The model under review builds one solid part; all positions refer to its coordinate system, in mm. Face numbers are marked on the shaded views. A direction names the side the tool comes from. Round coordinates to 2 decimals unless told otherwise and drop trailing zeros. Order: outer loops, then holes, each group sorted by start corner. A loop starts at its lowest first (then second) coordinate and runs counter-clockwise, first axis right, second up.
1) Clearance check with flat-ended pins moving along their axes: P1, Ø6, axis at x = -37.5, y = 103, coming from the +Z side; P2, Ø8, axis at x = 37.5, y = 103, coming from the +Z side; P3, Ø3, axis at x = 3, z = 33, coming from the -Y side. State where each tip first meets the part, or that it passes through.
2) To check wall thickness, follow L1, parallel to X at y = 8, z = 33.1; L2, parallel to X at y = 103, z = 18; L3, parallel to X at y = 132, z = 15.5. State the ranges of each line that lie inside material, in increasing order.
3) Consider section C-C (z = 7). Give the number of separate pieces and of enclosed holes in the cut face, then the cut area to 3 significant figures.
4) Machinability: for the marked faces 1, 2 and 3, which of the approach directions +Z, -Z, +X, -X, +Y, -Y give a long, thin tool a straight path to every point of the face, cutting with its end or side? Answer none if there is none.
5) Consider section A-A (x = 0). Give the boundary of the cut face in (y, z).
6) Consider section D-D (y = 118). Give the boundary of the cut face in (x, z).
7) Mouldability with a two-part tool opening along Y and no side actions: class the marked faces 4, 5, 6 and 7 as pulls with the +Y half, pulls with the -Y half, needs draft (parallel to the pull), parting line crosses it, or undercut.
8) Consider section B-B (y = 188). Give the boundary of the cut face in (x, z), then the cut area to 3 significant figures.
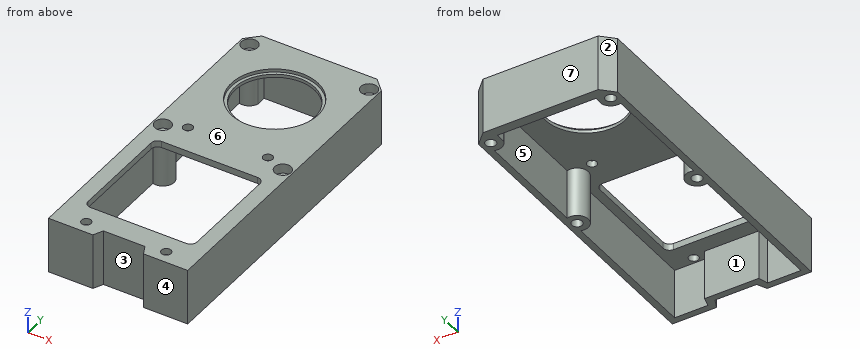
from build123d import *

# Parameters (mm, degrees)
SKETCH_R        = 3.25
SKETCH_R_2      = 3
SKETCH_R_3      = 25
PAD_DEPTH       = 35
POCKET_DEPTH    = 31
SKETCH003_R     = 5.1
POCKET001_DEPTH = 6
SKETCH004_R     = 27
POCKET002_DEPTH = 2


with BuildPart() as part:
    # Sketch → Pad (new body)
    with BuildSketch(Plane.XY):
        Polygon((-43.5, 190.5), (-43.5, 0), (-15.797846, 0), (-13, 6), (13, 6), (15.797846, 0), (43.5, 0), (43.5, 190.5), (36, 198), (-36, 198), align=None)
        with Locations((-37.5, 188)):
            Circle(SKETCH_R, mode=Mode.SUBTRACT)
        with Locations((37.5, 188)):
            Circle(SKETCH_R, mode=Mode.SUBTRACT)
        with Locations((-25, 108)):
            Circle(SKETCH_R_2, mode=Mode.SUBTRACT)
        with Locations((25, 108)):
            Circle(SKETCH_R_2, mode=Mode.SUBTRACT)
        with Locations((37.5, 103)):
            Circle(SKETCH_R, mode=Mode.SUBTRACT)
        with Locations((-37.5, 103)):
            Circle(SKETCH_R, mode=Mode.SUBTRACT)
        with Locations((-25, 8)):
            Circle(SKETCH_R_2, mode=Mode.SUBTRACT)
        with Locations((25, 8)):
            Circle(SKETCH_R_2, mode=Mode.SUBTRACT)
        with Locations((0, 154)):
            Circle(SKETCH_R_3, mode=Mode.SUBTRACT)
        with BuildLine():
            ThreePointArc((-30, 90), (-32.828431, 88.828423), (-34, 85.999989))
            Line((-34, 24), (-34, 85.999989))
            ThreePointArc((-34, 24), (-32.828427, 21.171573), (-30, 20))
            Line((-30, 20), (30, 20))
            ThreePointArc((30, 20), (32.828427, 21.171573), (34, 24))
            Line((34, 85.999989), (34, 24))
            ThreePointArc((34, 85.999989), (32.828431, 88.828424), (29.999999, 90))
            Line((-30, 90), (29.999999, 90))
        make_face(mode=Mode.SUBTRACT)
    extrude(amount=PAD_DEPTH)

    # Sketch002 → Pocket (cut)
    with BuildSketch(Plane(origin=(0, 0, 0), x_dir=(1, 0, 0), z_dir=(0, 0, -1))):
        with BuildLine():
            Line((-39.5, -96.291796), (-39.5, -4))
            Line((-39.5, -4), (-18.607695, -4))
            Line((-18.607695, -4), (-17, -10))
            Line((-17, -10), (17, -10))
            Line((17, -10), (18.607695, -4))
            Line((18.607695, -4), (39.5, -4))
            Line((39.5, -4), (39.5, -96.291796))
            ThreePointArc((39.5, -96.291796), (30.5, -103), (39.5, -109.708204))
            Line((39.5, -109.708204), (39.5, -181.291796))
            ThreePointArc((39.5, -181.291796), (34.170797, -181.84237), (30.791796, -186))
            Line((30.791796, -192), (30.791796, -186))
            Line((-30.791796, -192), (30.791796, -192))
            Line((-30.791796, -186), (-30.791796, -192))
            ThreePointArc((-30.791796, -186), (-34.170797, -181.84237), (-39.5, -181.291796))
            Line((-39.5, -109.708204), (-39.5, -181.291796))
            ThreePointArc((-39.5, -109.708204), (-30.5, -103), (-39.5, -96.291796))
        make_face()
    extrude(amount=-POCKET_DEPTH, mode=Mode.SUBTRACT)

    # Sketch003 → Pocket001 (cut)
    with BuildSketch(Plane.XY.offset(35)):
        with Locations((-37.371348, 188)):
            Circle(SKETCH003_R)
        with Locations((37.371348, 188)):
            Circle(SKETCH003_R)
        with Locations((-37.5, 103)):
            Circle(SKETCH003_R)
        with Locations((37.5, 103)):
            Circle(SKETCH003_R)
    extrude(amount=-POCKET001_DEPTH, mode=Mode.SUBTRACT)

    # Sketch004 → Pocket002 (cut)
    with BuildSketch(Plane.XY.offset(35)):
        with Locations((0, 154)):
            Circle(SKETCH004_R)
    extrude(amount=-POCKET002_DEPTH, mode=Mode.SUBTRACT)


solid = part.part
Answer below:
1. P1: passes through
1. P2: stops at z = 29
1. P3: stops at y = 6
2. L1: x = -43.5 to -28, -22 to 22, 28 to 43.5
2. L2: x = -43.5 to -40.75, -34.25 to -30.5, 30.5 to 34.25, 40.75 to 43.5
2. L3: x = -43.5 to -39.5, 39.5 to 43.5
3. separate pieces: 1
3. enclosed holes: 5
3. area: 2,610 mm2
4. face 1: -Z
4. face 2: +Z, -Z, -X, +Y
4. face 3: +Z, -Z, -Y
5. outline: (6, 0) - (10, 0) - (10, 31) - (20, 31) - (20, 35) - (6, 35) - close; (90, 31) - (129, 31) - (129, 33) - (127, 33) - (127, 35) - (90, 35) - close; (179, 31) - (192, 31) - (192, 0) - (198, 0) - (198, 35) - (181, 35) - (181, 33) - (179, 33) - close
6. outline: (-43.5, 0) - (-39.5, 0) - (-39.5, 31) - (39.5, 31) - (39.5, 0) - (43.5, 0) - (43.5, 35) - (-43.5, 35) - close
7. face 4: pulls with the -Y half
7. face 5: undercut
7. face 6: needs draft
7. face 7: pulls with the +Y half
8. outline: (-43.5, 0) - (-40.75, 0) - (-40.75, 29) - (-42.47, 29) - (-42.47, 35) - (-43.5, 35) - close; (-34.25, 0) - (-30.79, 0) - (-30.79, 31) - (30.79, 31) - (30.79, 0) - (34.25, 0) - (34.25, 29) - (32.27, 29) - (32.27, 35) - (-32.27, 35) - (-32.27, 29) - (-34.25, 29) - close; (40.75, 0) - (43.5, 0) - (43.5, 35) - (42.47, 35) - (42.47, 29) - (40.75, 29) - close
8. area: 637 mm2
